Autodesk Inventor part; units mm, degrees
ref_plane "YZ Plane" through (0, 0, 0) normal (1, 0, 0) x (0, 1, 0)
ref_plane "XZ Plane" through (0, 0, 0) normal (0, 1, 0) x (-1, 0, 0)
ref_plane "XY Plane" through (0, 0, 0) normal (0, 0, 1) x (1, 0, 0)
sketch "Sketch1" plane through (0, 0, 0) normal (0, 1, 0) x (-1, 0, 0)
  line L0 (9.5795, 5.4068) -> (9.4722, -5.5927)
  line L1 (9.4722, -5.5927) -> (-0.1073, -10.9995)
  line L2 (-0.1073, -10.9995) -> (-9.5795, -5.4068)
  line L3 (-9.5795, -5.4068) -> (-9.4722, 5.5927)
  line L4 (-9.4722, 5.5927) -> (0.1073, 10.9995)
  line L5 (0.1073, 10.9995) -> (9.5795, 5.4068)
  circle A0 centre (0, 0) radius 6
  circle A1 centre (0, 0) radius 9
  dimension "d0" = 11
  dimension "d1" = 12
  dimension "d8" = 18
extrude "Extrusion1" add sketch "Sketch1" along normal blind 8 contours L0 L1 L2 L3 L4 L5 | A1
extrude "Extrusion2" add sketch "Sketch1" against normal blind 4 contours A1
fillet "Fillet1" radius 2 1 edges at (9, -4, 0)
chamfer "Chamfer1" distance 1 angle 45 1 edges at (9, 0, 0)
thread "Thread1"
chamfer "Chamfer2" distance 1 angle 45 2 edges at (6, -4, 0) (6, 8, 0)
fillet "Fillet3" radius 1 6 edges at (-9.5795, 4, 5.4068) (-9.4722, 4, -5.5927) (0.1073, 4, -10.9995) (-0.1073, 4, 10.9995) (9.4722, 4, 5.5927) (9.5795, 4, -5.4068)
fillet "Fillet4" radius 0.3 12 edges at (9.339, 8, 5.514) (9.5258, 8, 0.0929) (9.4448, 8, -5.3308) (4.8434, 8, -8.2031) (0.1058, 8, -10.8448) (-4.6824, 8, -8.2961) (-9.339, 8, -5.514) (-9.5258, 8, -0.0929) (-9.4448, 8, 5.3308) (-4.8434, 8, 8.2031) (-0.1058, 8, 10.8448) (4.6824, 8, 8.2961)
properties part number "SpanoloAnya"
Here's how the part is built. I have some questions about the finished solid (model axes, mm). A direction names the side the tool comes from. Coordinates: 2 decimals unless noted, no trailing zeros. Order: outer loops, then holes, each group sorted by start corner. A loop starts at its lowest first (then second) coordinate and runs counter-clockwise, first axis right, second up.
Item 1: For P1, Ø0.9, axis at x = 0.5, z = 10.5, coming from the -Y side; P2, Ø3, axis at x = 3, z = -3, coming from the +Y side; P3, Ø0.6, axis at x = -9, z = -4.5, coming from the -Y side; P4, Ø1.1, axis at x = 8.5, z = 5, coming from the -Y side, each with a flat end and sliding along its axis, tell me the tip position at first contact or that it passes through.
Result sheet:
P1: stops at y = 0
P2: passes through
P3: stops at y = -0.24
P4: stops at y = -0.69
Item 2: I need wall thicknesses on line 1 (Z direction, x = 0, y = 3.25); line 2 (Z direction, x = 4, y = -2); line 3 (X direction, y = 3.75, z = -3.5). Which ranges of each line are inside material? Lowest first, please.
Result sheet:
line 1: z = -10.84 to -6, 6 to 10.84
line 2: z = -8.06 to -4.47, 4.47 to 8.06
line 3: x = -9.49 to -4.87, 4.87 to 9.56
Item 3: If we section it at B-B on y = -1.5: List the corners of the cut face in (x, z) for me, plus the area to 3 significant figures.
Result sheet:
outline: circle Ø18 at (0, 0); hole circle Ø12 at (0, 0)
area: 141 mm2
Item 4: For faces 1 (the face through (1.172, -1.493, 8.923)), 2 (the face through (-9, 0, 5)), 3 (the face through (9.335, 3.904, 5.52)), 4 (the face through (-9, 0, -5)), 5 (the face through (9, 0, 5)), which set-ups out of +Z, -Z, +X, -X, +Y, -Y let a thin tool reach every point of the face, with its end or its side?
Result sheet:
face 1: -Y
face 2: +Z, -X, -Y
face 3: +Z, +X, +Y, -Y
face 4: -Z, -X, -Y
face 5: +Z, +X, -Y
Item 5: If we section it at A-A on y = 6.25: List the corners of the cut face in (x, z) for me, plus the area to 3 significant figures.
Result sheet:
outline: (-9.57, 4.83) - (-9.48, -5.02) arc R1 ccw to (-8.97, -5.88) - (-0.4, -10.72) arc R1 ccw to (0.6, -10.71) - (9.08, -5.7) arc R1 ccw to (9.57, -4.83) - (9.48, 5.02) arc R1 ccw to (8.97, 5.88) - (0.4, 10.72) arc R1 ccw to (-0.6, 10.71) - (-9.08, 5.7) arc R1 ccw to start; hole circle Ø12 at (0, 0)
area: 201 mm2
